For this review, take the finished solid that the model builds, in its own axes (mm). A direction names the side the tool comes from. Give positions to 0.01 mm unless a question says otherwise; leave off trailing zeros. Order: outer loops, then holes, each group sorted by start corner. A loop starts at its lowest first (then second) coordinate and runs counter-clockwise, first axis right, second up. Notation, with made-up numbers: (36.5, -32) -> (81.5, -32) arc R16 ccw to (81.5, -14) -> close; hole circle Ø7 at (84.5, 72.5). An arc over 180 degrees is marked (long way). One line per item, written item: value. Start each with the question number.
Autodesk Inventor part; units mm, degrees
ref_plane "YZ Plane" through (0, 0, 0) normal (1, 0, 0) x (0, 1, 0)
ref_plane "XZ Plane" through (0, 0, 0) normal (0, 1, 0) x (-1, 0, 0)
ref_plane "XY Plane" through (0, 0, 0) normal (0, 0, 1) x (1, 0, 0)
sketch "Sketch1" plane through (0, 0, 0) normal (0, 0, 1) x (1, 0, 0)
  circle A0 centre (0, 0) radius 35
  circle A1 centre (0, 0) radius 28
  dimension "d0" = 70
  dimension "d1" = 56
extrude "Extrusion1" add sketch "Sketch1" along normal blind 210
sketch "Sketch2" plane through (0, 0, 0) normal (0, 0, -1) x (-1, 0, 0)
  circle A0 centre (0, 0) radius 31.5
extrude "Extrusion2" add sketch "Sketch2" against normal blind 7
sketch "Sketch3" plane through (0, 0, 210) normal (0, 0, 1) x (1, 0, 0)
  circle A0 centre (0, 0) radius 35
  line L0 (35, 0) -> (17.5, -30.3109)
  line L1 (17.5, -30.3109) -> (-17.5, -30.3109)
  line L2 (-17.5, -30.3109) -> (-35, 0)
  line L3 (-35, 0) -> (-17.5, 30.3109)
  line L4 (-17.5, 30.3109) -> (17.5, 30.3109)
  line L5 (17.5, 30.3109) -> (35, 0)
  line L6 (-17.5, 30.3109) -> (17.5, -30.3109)
  line L7 (-17.5, -30.3109) -> (17.5, 30.3109)
  line L8 (-35, 0) -> (35, 0)
  line L9 (-17.5, 30.3109) -> (-15.5, 26.8468)
  line L10 (17.5, 30.3109) -> (15.5, 26.8468)
  line L11 (35, 0) -> (31, 0)
  line L12 (17.5, -30.3109) -> (15.5, -26.8468)
  line L13 (-17.5, -30.3109) -> (-15.5, -26.8468)
  line L14 (-35, 0) -> (-31, 0)
  dimension "d6" = 4
  dimension "d7" = 4
  dimension "d8" = 4
  dimension "d9" = 4
  dimension "d10" = 4
  dimension "d11" = 4
hole "Hole1" at (-15.5, 26.8468, 210) at (-31, 0, 210) at (-15.5, -26.8468, 210) at (15.5, 26.8468, 210) at (31, 0, 210) at (15.5, -26.8468, 210) direction (0, 0, -1) diameter 3 depth 8 tip angle 118
properties part number "battery_Tube"
Q1. For line 1 along Y through (x, z) = (-0.5, 65); line 2 along Z through (x, y) = (17, 16); line 3 along Y through (x, z) = (15.5, 207), list the stretches that pass through material, from the lowest coordinate up.
Q2. Take a section at A-A (x = 19). State the section outline as (y, z) points, and give its area (3 significant figures).
Q3. For faces 4 (the flat face through (0, 0, 0)), 5 (the flat face through (0, 0, 7)), list the 3-axis set-ups (+Z, -Z, +X, -X, +Y, -Y) from which the entire face can be reached by the end or side of a thin tool; tool diameter is ignored.
Q4. Take a section at C-C (z = 175). State the section outline as (x, y) points, and give its area (3 significant figures).
Q5. For pin 1 Ø5 at (y, z) = (-5, 180) entering from -X; pin 2 Ø10 at (x, y) = (8, -16) entering from +Z; pin 3 Ø3.5 at (x, y) = (15.5, -26.85) entering from -Z; pin 4 Ø1.8 at (x, y) = (-31, 0) entering from +Z, all flat-tipped, find the tip position at first contact; note any pin that passes through.
Q6. Take a section at B-B (y = 6.5). State the section outline as (x, z) points.
Q7. Mouldability with a two-part tool opening along X and no side actions: class faces 1 (the cylindrical face through (-28, 21, 104)), 2 (the cylindrical face through (25.865, 10.724, 107.079)), 3 (the flat face through (-15.7, 23.5, 210)) as pulls with the +X half, pulls with the -X half, needs draft (parallel to the pull), parting line crosses it, or undercut.
Answers below:
1. line 1: y = -35 to -28, 28 to 35
1. line 2: z = 0 to 7
1. line 3: y = -31.38 to -28.35, -25.35 to -23.32, 23.32 to 25.35, 28.35 to 31.38
2. outline: (-29.39, 0) -> (29.39, 0) -> (29.39, 210) -> (20.57, 210) -> (20.57, 7) -> (-20.57, 7) -> (-20.57, 210) -> (-29.39, 210) -> close
2. area: 4,000 mm²
3. face 4: -Z, +X, -X, +Y, -Y
3. face 5: +Z
4. outline: circle Ø70 at (0, 0); hole circle Ø56 at (0, 0)
4. area: 1,390 mm²
5. pin 1: stops at x = -34.91
5. pin 2: stops at z = 7
5. pin 3: stops at z = 0
5. pin 4: stops at z = 201.64
6. outline: (-34.39, 0) -> (34.39, 0) -> (34.39, 210) -> (27.24, 210) -> (27.24, 7) -> (-27.24, 7) -> (-27.24, 210) -> (-34.39, 210) -> close
7. face 1: parting line crosses it
7. face 2: undercut
7. face 3: needs draft
